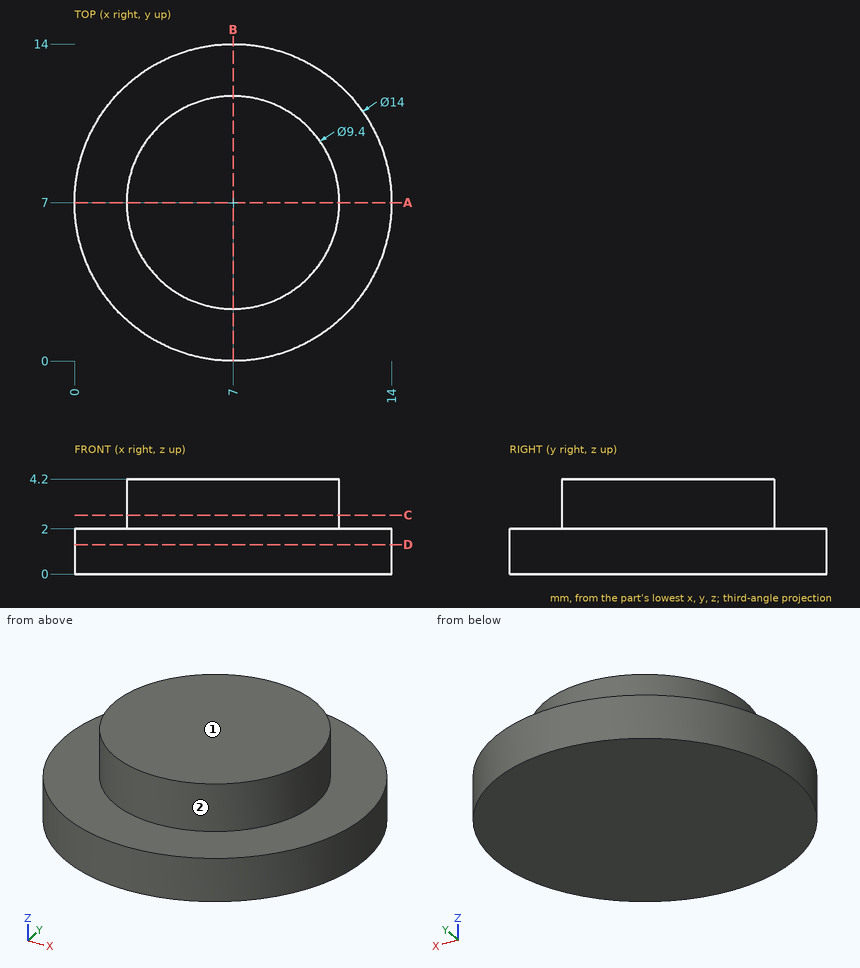
For this review, use the dimensioned drawing (mm, ordinates from the lowest corner) and the shaded views. A direction names the side the tool comes from. Give positions to 0.01 mm unless a question says otherwise; leave off trailing zeros. Loops run counter-clockwise (first coordinate to the right, second up) from the corner with the lowest first, then second, coordinate; pieces in that order, holes last.
Item 1: Insertion check: pin 1 (2 mm diameter, centred on y = 10.5, z = 0.5, fed in from +X); pin 2 (2 mm diameter, centred on x = 6, z = 0.5, fed in from +Y). Each pin has a flat end and moves straight along its axis. Give the tip position at first contact, or say it passes through.
Item 2: Take a section at C-C, the plane z = 2.6. State the section outline as (x, y) points.
Item 3: Tool access review of the marked faces 1 and 2: name each direction out of +Z, -Z, +X, -X, +Y, -Y from which nothing blocks a thin tool from reaching the whole face with its end or side.
Item 4: For line 1 along Z through (x, y) = (13, 6.25); line 2 along X through (y, z) = (4.75, 0.9); line 3 along X through (y, z) = (5.5, 2.05), list the stretches that pass through material, from the lowest coordinate up.
Item 5: Take a section at D-D, the plane z = 1.3. State the section outline as (x, y) points.
Item 6: Take a section at A-A, the plane y = 7. State the section outline as (x, z) points, and give its area (3 significant figures).
Calculated:
1. pin 1: stops at x = 13.54
1. pin 2: stops at y = 14
2. outline: circle Ø9.4 at (7, 7)
3. face 1: +Z, +X, -X, +Y, -Y
3. face 2: +Z
4. line 1: z = 0 to 2
4. line 2: x = 0.37 to 13.63
4. line 3: x = 2.55 to 11.45
5. outline: circle Ø14 at (7, 7)
6. outline: (0, 0) - (14, 0) - (14, 2) - (11.7, 2) - (11.7, 4.2) - (2.3, 4.2) - (2.3, 2) - (0, 2) - close
6. area: 48.7 mm2
